from build123d import *

# Parameters (mm, degrees)
BOSS_EXTRUDE1_DEPTH = 10


with BuildPart() as part:
    # Sketch1 → Boss-Extrude1 (new body)
    with BuildSketch(Plane(origin=(0, 0, 0), x_dir=(1, 0, 0), z_dir=(0, 1, 0))):
        with BuildLine():
            Line((-0.77475919, 17.805575817), (-0.77475919, 18.205472922))
            Line((-0.77475919, 18.205472922), (-2.591328104, 16.388904008))
            Line((-2.591328104, 16.388904008), (-2.591328104, 15.751300349))
            Line((-2.591328104, 15.751300349), (-2.362753208, 15.246029526))
            Line((-2.362753208, 15.246029526), (-2.591328104, 15.017454629))
            Line((-2.591328104, 15.017454629), (-5.779346397, 18.205472922))
            Line((-5.779346397, 18.205472922), (-6.095268046, 18.892889731))
            Line((-6.095268046, 18.892889731), (-12.218826377, 15.246029526))
            add(Edge.make_bspline(
                [(-12.218826377, 15.246029526), (-11.778721685, 20.620695324), (-8.581947184, 24.333309757)],
                knots=[0, 0, 0, 1, 1, 1], degree=2))
            Line((-8.581947184, 24.333309757), (-9.157047212, 24.259356466))
            add(Edge.make_bspline(
                [(-9.157047212, 24.259356466), (-14.447655818, 18.459017457), (-14.037673367, 11.71891231)],
                knots=[0, 0, 0, 1, 1, 1], degree=2))
            Line((-14.037673367, 11.71891231), (-6.606809824, 16.748676517))
            add(Edge.make_bspline(
                [(-6.606809824, 16.748676517), (-4.84160761, 15.196820639), (-2.713996128, 14.373140945)],
                knots=[0, 0, 0, 1, 1, 1], degree=2))
            Line((-2.713996128, 14.373140945), (-3.022885214, 14.011805458))
            Line((-3.022885214, 14.011805458), (-7.04843704, 15.185986651))
            Line((-7.04843704, 15.185986651), (-16.542260828, 8.414995079))
            Line((-16.542260828, 8.414995079), (-16.750184267, 8.475642613))
            Line((-16.750184267, 8.475642613), (-16.844000716, 8.999446115))
            add(Edge.make_bspline(
                [(-16.844000716, 8.999446115), (-17.398318859, 14.288056659), (-15.498292646, 18.892889731)],
                knots=[0, 0, 0, 0.937492037, 0.937492037, 0.937492037], degree=2))
            Line((-15.498292646, 18.892889731), (-15.498292646, 19.083480243))
            Line((-15.498292646, 19.083480243), (-16.018185643, 18.698181665))
            add(Edge.make_bspline(
                [(-16.018185643, 18.698181665), (-19.54860855, 11.964227915), (-17.772645014, 5.545401207)],
                knots=[0, 0, 0, 1, 1, 1], degree=2))
            Line((-17.772645014, 5.545401207), (-6.976425445, 13.546601594))
            Line((-6.976425445, 13.546601594), (-3.220749094, 13.546601594))
            Line((-3.220749094, 13.546601594), (-3.220749094, 12.787927187))
            Line((-3.220749094, 12.787927187), (-7.04843704, 12.523140875))
            add(Edge.make_bspline(
                [(-7.04843704, 12.523140875), (-11.378277138, 6.786058759), (-17.368277161, 3.344273399)],
                knots=[0, 0, 0, 1, 1, 1], degree=2))
            add(Edge.make_bspline(
                [(-17.368277161, 3.344273399), (-15.724066268, -8.863327627), (-9.366664211, -18.723496609)],
                knots=[0, 0, 0, 0.983877667, 0.983877667, 0.983877667], degree=2))
            Line((-9.366664211, -18.723496609), (-8.360846592, -20.115700618))
            Line((-8.360846592, -20.115700618), (-8.984631154, -18.211516166))
            add(Edge.make_bspline(
                [(-8.984631154, -18.211516166), (-13.367422275, -8.565356306), (-14.632198794, 1.702238546)],
                knots=[0, 0, 0, 0.96561084, 0.96561084, 0.96561084], degree=2))
            Line((-14.632198794, 1.702238546), (-6.095268046, 11.245692572))
            Line((-6.095268046, 11.245692572), (-3.220749094, 12.334656835))
            Line((-3.220749094, 12.334656835), (-3.137312332, 11.517506569))
            Line((-3.137312332, 11.517506569), (-5.68828216, 10.551113575))
            add(Edge.make_bspline(
                [(-5.68828216, 10.551113575), (-8.289822739, 5.230431142), (-11.398307003, 0.207327452)],
                knots=[0, 0, 0, 0.941866113, 0.941866113, 0.941866113], degree=2))
            add(Edge.make_bspline(
                [(-11.398307003, 0.207327452), (-9.259704318, -11.446844699), (-4.663293434, -22.207552312)],
                knots=[0, 0, 0, 0.984459997, 0.984459997, 0.984459997], degree=2))
            Line((-4.663293434, -22.207552312), (-3.52644295, -23.884260193))
            Line((-3.52644295, -23.884260193), (-4.094868192, -21.920639742))
            add(Edge.make_bspline(
                [(-4.094868192, -21.920639742), (-7.201743798, -11.767427454), (-8.842724338, -1.332659634)],
                knots=[0, 0, 0, 0.95775591, 0.95775591, 0.95775591], degree=2))
            Line((-8.842724338, -1.332659634), (-8.901419383, -0.55237788))
            Line((-8.901419383, -0.55237788), (-4.663293434, 9.459890703))
            Line((-4.663293434, 9.459890703), (-3.137312332, 10.808717055))
            Line((-3.137312332, 10.808717055), (-2.918598052, 10.825169375))
            Line((-2.918598052, 10.825169375), (-2.254002061, 9.809392881))
            Line((-2.254002061, 9.809392881), (-4.219363172, 7.408826128))
            add(Edge.make_bspline(
                [(-4.219363172, 7.408826128), (-4.079064375, 3.638553555), (-3.236682616, 0)],
                knots=[0, 0, 0, 0.892205795, 0.892205795, 0.892205795], degree=2))
            add(Edge.make_bspline(
                [(-3.236682616, 0), (-2.55670829, -2.640008962), (-1.031376318, -4.773443308)],
                knots=[0, 0, 0, 0.876843131, 0.876843131, 0.876843131], degree=2))
            add(Edge.make_bspline(
                [(-1.031376318, -4.773443308), (-0.582556801, -4.206513749), (0, -4.327217184)],
                knots=[0, 0, 0, 1, 1, 1], degree=2))
            add(Edge.make_bspline(
                [(1.031376318, -4.773443308), (0.582556801, -4.206513749), (0, -4.327217184)],
                knots=[0, 0, 0, 1, 1, 1], degree=2))
            add(Edge.make_bspline(
                [(3.236682616, 0), (2.55670829, -2.640008962), (1.031376318, -4.773443308)],
                knots=[0, 0, 0, 0.876843131, 0.876843131, 0.876843131], degree=2))
            add(Edge.make_bspline(
                [(4.219363172, 7.408826128), (4.079064375, 3.638553555), (3.236682616, 0)],
                knots=[0, 0, 0, 0.892205795, 0.892205795, 0.892205795], degree=2))
            Line((4.219363172, 7.408826128), (2.254002061, 9.809392881))
            Line((2.254002061, 9.809392881), (2.918598052, 10.825169375))
            Line((2.918598052, 10.825169375), (3.137312332, 10.808717055))
            Line((3.137312332, 10.808717055), (4.663293434, 9.459890703))
            Line((4.663293434, 9.459890703), (8.901419383, -0.55237788))
            Line((8.901419383, -0.55237788), (8.842724338, -1.332659634))
            add(Edge.make_bspline(
                [(4.094868192, -21.920639742), (7.201743798, -11.767427454), (8.842724338, -1.332659634)],
                knots=[0, 0, 0, 0.95775591, 0.95775591, 0.95775591], degree=2))
            Line((4.094868192, -21.920639742), (3.52644295, -23.884260193))
            Line((3.52644295, -23.884260193), (4.663293434, -22.207552312))
            add(Edge.make_bspline(
                [(11.398307003, 0.207327452), (9.259704318, -11.446844699), (4.663293434, -22.207552312)],
                knots=[0, 0, 0, 0.984459997, 0.984459997, 0.984459997], degree=2))
            add(Edge.make_bspline(
                [(5.68828216, 10.551113575), (8.289822739, 5.230431142), (11.398307003, 0.207327452)],
                knots=[0, 0, 0, 0.941866113, 0.941866113, 0.941866113], degree=2))
            Line((5.68828216, 10.551113575), (3.137312332, 11.517506569))
            Line((3.137312332, 11.517506569), (3.220749094, 12.334656835))
            Line((3.220749094, 12.334656835), (6.095268046, 11.245692572))
            Line((6.095268046, 11.245692572), (14.632198794, 1.702238546))
            add(Edge.make_bspline(
                [(8.984631154, -18.211516166), (13.367422275, -8.565356306), (14.632198794, 1.702238546)],
                knots=[0, 0, 0, 0.96561084, 0.96561084, 0.96561084], degree=2))
            Line((8.984631154, -18.211516166), (8.360846592, -20.115700618))
            Line((8.360846592, -20.115700618), (9.366664211, -18.723496609))
            add(Edge.make_bspline(
                [(17.368277161, 3.344273399), (15.724066268, -8.863327627), (9.366664211, -18.723496609)],
                knots=[0, 0, 0, 0.983877667, 0.983877667, 0.983877667], degree=2))
            add(Edge.make_bspline(
                [(7.04843704, 12.523140875), (11.378277138, 6.786058759), (17.368277161, 3.344273399)],
                knots=[0, 0, 0, 1, 1, 1], degree=2))
            Line((7.04843704, 12.523140875), (3.220749094, 12.787927187))
            Line((3.220749094, 12.787927187), (3.220749094, 13.546601594))
            Line((3.220749094, 13.546601594), (6.976425445, 13.546601594))
            Line((6.976425445, 13.546601594), (17.772645014, 5.545401207))
            add(Edge.make_bspline(
                [(16.018185643, 18.698181665), (19.54860855, 11.964227915), (17.772645014, 5.545401207)],
                knots=[0, 0, 0, 1, 1, 1], degree=2))
            Line((16.018185643, 18.698181665), (15.498292646, 19.083480243))
            Line((15.498292646, 19.083480243), (15.498292646, 18.892889731))
            add(Edge.make_bspline(
                [(16.844000716, 8.999446115), (17.398318859, 14.288056659), (15.498292646, 18.892889731)],
                knots=[0, 0, 0, 0.937492037, 0.937492037, 0.937492037], degree=2))
            Line((16.844000716, 8.999446115), (16.750184267, 8.475642613))
            Line((16.750184267, 8.475642613), (16.542260828, 8.414995079))
            Line((16.542260828, 8.414995079), (7.04843704, 15.185986651))
            Line((7.04843704, 15.185986651), (3.022885214, 14.011805458))
            Line((3.022885214, 14.011805458), (2.713996128, 14.373140945))
            add(Edge.make_bspline(
                [(6.606809824, 16.748676517), (4.84160761, 15.196820639), (2.713996128, 14.373140945)],
                knots=[0, 0, 0, 1, 1, 1], degree=2))
            Line((6.606809824, 16.748676517), (14.037673367, 11.71891231))
            add(Edge.make_bspline(
                [(9.157047212, 24.259356466), (14.447655818, 18.459017457), (14.037673367, 11.71891231)],
                knots=[0, 0, 0, 1, 1, 1], degree=2))
            Line((9.157047212, 24.259356466), (8.581947184, 24.333309757))
            add(Edge.make_bspline(
                [(12.218826377, 15.246029526), (11.778721685, 20.620695324), (8.581947184, 24.333309757)],
                knots=[0, 0, 0, 1, 1, 1], degree=2))
            Line((12.218826377, 15.246029526), (6.095268046, 18.892889731))
            Line((6.095268046, 18.892889731), (5.779346397, 18.205472922))
            Line((5.779346397, 18.205472922), (2.591328104, 15.017454629))
            Line((2.591328104, 15.017454629), (2.362753208, 15.246029526))
            Line((2.362753208, 15.246029526), (2.591328104, 15.751300349))
            Line((2.591328104, 15.751300349), (2.591328104, 16.388904008))
            Line((2.591328104, 16.388904008), (0.77475919, 18.205472922))
            Line((0.77475919, 18.205472922), (0.77475919, 17.805575817))
            add(Edge.make_bspline(
                [(0.77475919, 17.805575817), (1.570165167, 16.532957411), (1.031376318, 15.489501362)],
                knots=[0, 0, 0, 1, 1, 1], degree=2))
            Line((1.031376318, 15.489501362), (-1.031376318, 15.489501362))
            add(Edge.make_bspline(
                [(-0.77475919, 17.805575817), (-1.570165167, 16.532957411), (-1.031376318, 15.489501362)],
                knots=[0, 0, 0, 1, 1, 1], degree=2))
        make_face()
    extrude(amount=BOSS_EXTRUDE1_DEPTH)


solid = part.part
The listing builds one solid part. Answer for the finished solid, in the listing's coordinates (mm). A direction names the side the tool comes from. Give positions to 0.01 mm unless a question says otherwise; leave off trailing zeros. Write each question's results on one line, items separated by ' | '.
1. Consider probe 1 along X at (y, z) = (1.25, 0.5); probe 2 along X at (y, z) = (6.75, -2); probe 3 along X at (y, z) = (2.25, 8). Determine where each line is inside the solid, lowest interval first. Write a range as from..to.
Resolved:
probe 1: x = -16.72..-14.32, -11.27..-8.88, -3.1..3.1, 8.88..11.27, 14.32..16.72 | probe 2: x = -17.17..-14.37, -10.31..-7.82, -3.64..3.64, 7.82..10.31, 14.37..17.17 | probe 3: x = -14.65..-12.7, -9.56..-7.64, 7.64..9.56, 12.7..14.65
2. For a pull along X with two mould halves and no side action, classify faces 4 (the face through (8.857, 4.93, 19.429)), 5 (the face through (4.208, 4.93, -16.634)), 6 (the face through (8.677, 4.93, 19.15)), 7 (the face through (-4.103, 4.93, 23.034)) as +X half, -X half, draft (parallel to the pull), parting line (faces both ways), or undercut.
Resolved:
face 4: +X half | face 5: undercut | face 6: undercut | face 7: -X half
3. Which of the six approach directions +Z, -Z, +X, -X, +Y, -Y give full straight-line access (tool end or side, diameter ignored) to faces 1 (the face through (3.815, 4.93, 22.889)), 2 (the face through (1.7, 4.93, -17.28)), 3 (the face through (-8.87, 4.93, 19.41))?
Resolved:
face 1: +Y, -Y | face 2: -Z, +Y, -Y | face 3: +Z, -X, +Y, -Y
4. Flat-ended cylindrical pins translate along their axes: P1, Ø0.7, axis at y = 4.5, z = -16, coming from the -X side; P2, Ø1.5, axis at x = -7, y = 2, coming from the -Z side; P3, Ø0.6, axis at y = 3, z = -13, coming from the +X side. Find the tip coordinate at first contact, or state that the pin passes through.
Resolved:
P1: stops at x = -17.35 | P2: stops at z = -18.8 | P3: stops at x = 18.12
5. Find section A-A, the plane x = 13. Count the separate pieces of the cut face and the enclosed holes in it, then the cut area to 3 significant figures.
Resolved:
separate pieces: 4 | enclosed holes: 0 | area: 157 mm^2
